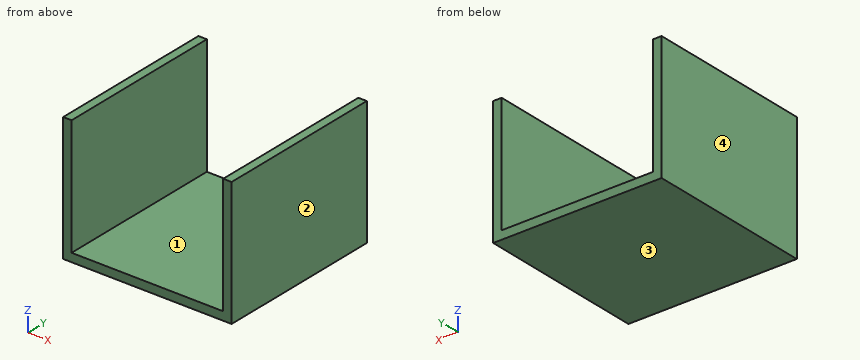
```python
from build123d import *

# Parameters (mm, degrees)
SKETCH1_W           = 100
SKETCH1_H           = 100
BOSS_EXTRUDE1_DEPTH = 5
SKETCH2_W           = 5
SKETCH2_H           = 100
BOSS_EXTRUDE3_DEPTH = 70


with BuildPart() as part:
    # Sketch1 → Boss-Extrude1 (new body)
    with BuildSketch(Plane.XY):
        Rectangle(SKETCH1_W, SKETCH1_H)
    extrude(amount=-BOSS_EXTRUDE1_DEPTH)

    # Sketch2 → Boss-Extrude3 (add)
    with BuildSketch(Plane.XY):
        with Locations((-47.5, 0)):
            Rectangle(SKETCH2_W, SKETCH2_H)
        with Locations((47.5, 0)):
            Rectangle(SKETCH2_W, SKETCH2_H)
    extrude(amount=BOSS_EXTRUDE3_DEPTH)


solid = part.part
```
Work out the finished part from the listing and answer in its coordinate system (mm). Face numbers are marked on the shaded views. Give positions to 0.01 mm unless a question says otherwise; leave off trailing zeros. Loops run counter-clockwise (first coordinate to the right, second up) from the corner with the lowest first, then second, coordinate; pieces in that order, holes last. Notation, with made-up numbers: (4, 78) - (21, 78) arc R27 ccw to (21, 107) - close; hole circle Ø10 at (-13.75, 33.5). An arc over 180 degrees is marked (long way). Use CSV: the item, a comma, the result in double quotes. Start each with the question number.
(1) Determine the mould class of the marked faces 1, 2, 3 and 4 for opening direction X: released by +X, released by -X, zero draft, split by the parting line, or undercut.
(2) Find the intervals of material crossed by L1, parallel to X at y = 18, z = 17; L2, parallel to Z at x = 40, y = 39, in increasing order.
(3) Find section A-A, the plane z = 8. Determine the outline of the cut face in (x, y).
(4) Find section C-C, the plane x = -23.5. Determine the outline of the cut face in (y, z), plus the area to 3 significant figures.
(5) This flat-tipped pin is pushed along its axis until it touches: pin 1 (4 mm diameter, centred on x = -5, y = -25.5, fed in from +Z). Where does it stop, or does it pass through?
(6) Find section B-B, the plane y = 33. Determine the outline of the cut face in (x, z), plus the area to 3 significant figures.
Results found:
1,face 1,"undercut"
1,face 2,"released by +X"
1,face 3,"zero draft"
1,face 4,"released by -X"
2,L1,"-50 to -45, 45 to 50"
2,L2,"-5 to 0"
3,outline,"(-50, -50) - (-45, -50) - (-45, 50) - (-50, 50) - close; (45, -50) - (50, -50) - (50, 50) - (45, 50) - close"
4,outline,"(-50, -5) - (50, -5) - (50, 0) - (-50, 0) - close"
4,area,"500 mm^2"
5,pin 1,"z = 0"
6,outline,"(-50, -5) - (50, -5) - (50, 70) - (45, 70) - (45, 0) - (-45, 0) - (-45, 70) - (-50, 70) - close"
6,area,"1,200 mm^2"
